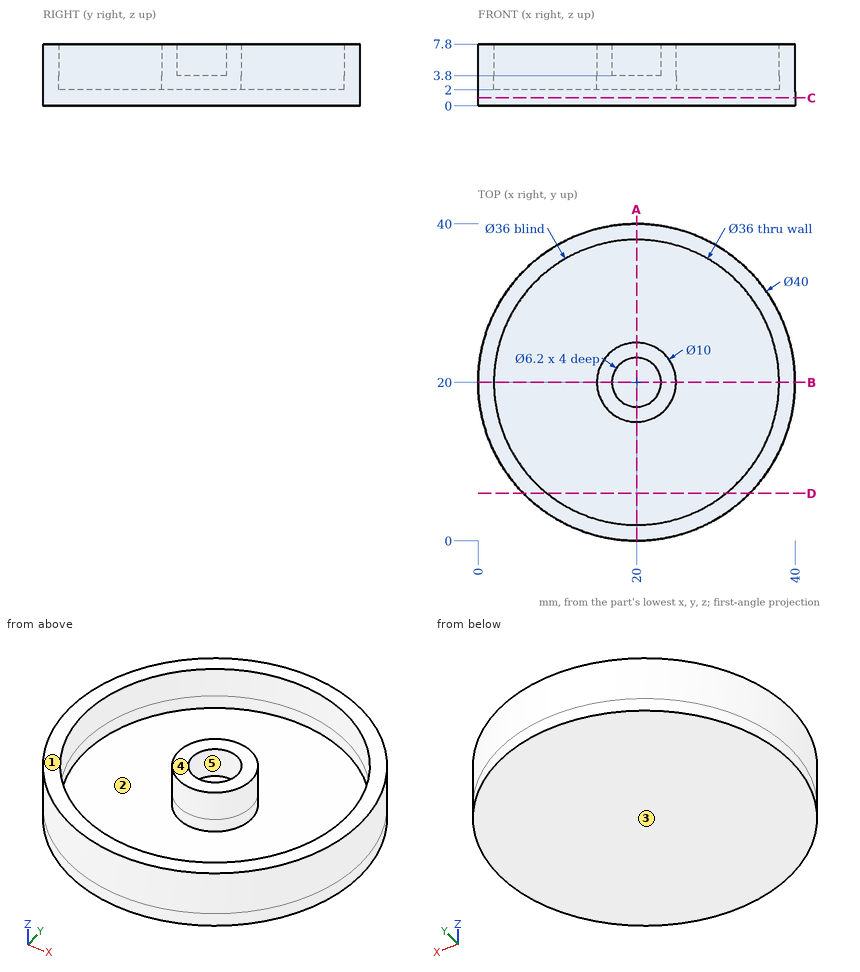
Answer from the drawing. Dimensions are ordinates in mm from the lowest x, y and z of the part. A direction names the side the tool comes from. Coordinates: 2 decimals unless noted, no trailing zeros. Order: outer loops, then holes, each group sorted by start corner. A loop starts at its lowest first (then second) coordinate and runs counter-clockwise, first axis right, second up. Notation, with made-up numbers: (21, -12.75) - (57, -12.75) arc R13 cw to (57, 10.25) - close; hole circle Ø8 at (-24.5, -11.5). An arc over 180 degrees is marked (long way). Put each result on its own line as item: value. Start each with the question number.
1) For a pull along Z with two mould halves and no side action, classify the marked faces 3, 4 and 5 as released by +Z, released by -Z, zero draft, split by the parting line, or undercut.
2) Find section D-D (y = 6). Give the vertices of the cut face in (x, z).
3) Find section C-C (z = 1). Give the vertices of the cut face in (x, y).
4) Find section A-A (x = 20). Give the vertices of the cut face in (y, z).
5) Flat-ended cylindrical pins translate along their axes: pin 1 (5 mm diameter, centred on x = 20, y = 20.5, fed in from +Z); pin 2 (4 mm diameter, centred on x = 23, z = 2.5, fed in from -Y) (3 decimals); pin 3 (3 mm diameter, centred on x = 35, z = 6, fed in from +Y). Find the tip coordinate at first contact, or state that the pin passes through.
6) Find the intervals of material crossed by line 1 (Y direction, x = 20, z = 5.4); line 2 (Y direction, x = 20, z = 3.1); line 3 (Y direction, x = 17, z = 3.75), in increasing order. Write a range as from..to.
7) For the marked faces 1 and 2, determine the directions among +Z, -Z, +X, -X, +Y, -Y from which every point of the face is accessible in a straight line to the end or side of a thin tool.
Results list:
1. face 3: released by -Z
1. face 4: released by +Z
1. face 5: zero draft
2. outline: (5.72, 0) - (34.28, 0) - (34.28, 7.8) - (31.31, 7.8) - (31.31, 2) - (8.69, 2) - (8.69, 7.8) - (5.72, 7.8) - close
3. outline: circle Ø40 at (20, 20)
4. outline: (0, 0) - (40, 0) - (40, 7.8) - (38, 7.8) - (38, 2) - (25, 2) - (25, 7.8) - (23.1, 7.8) - (23.1, 3.8) - (16.9, 3.8) - (16.9, 7.8) - (15, 7.8) - (15, 2) - (2, 2) - (2, 7.8) - (0, 7.8) - close
5. pin 1: stops at z = 3.8
5. pin 2: stops at y = 0.025
5. pin 3: stops at y = 34.76
6. line 1: y = 0..2, 15..16.9, 23.1..25, 38..40
6. line 2: y = 0..2, 15..25, 38..40
6. line 3: y = 0.23..2.25, 16..24, 37.75..39.77
7. face 1: +Z, +X, -X, +Y, -Y
7. face 2: +Z
